Source: CAD feature listing. Evaluate the final solid. Frame: model axes, mm. Face numbers are marked on the shaded views. A direction names the side the tool comes from. Give positions to 0.01 mm unless a question says otherwise; leave off trailing zeros. Order: outer loops, then holes, each group sorted by start corner. A loop starts at its lowest first (then second) coordinate and runs counter-clockwise, first axis right, second up. Notation, with made-up numbers: (-24, -14.5) -> (21, -14.5) arc R15 ccw to (21, -5.5) -> close; hole circle Ø9 at (26.25, 22). An arc over 180 degrees is marked (long way). Answer in a Markdown table with one row per item.
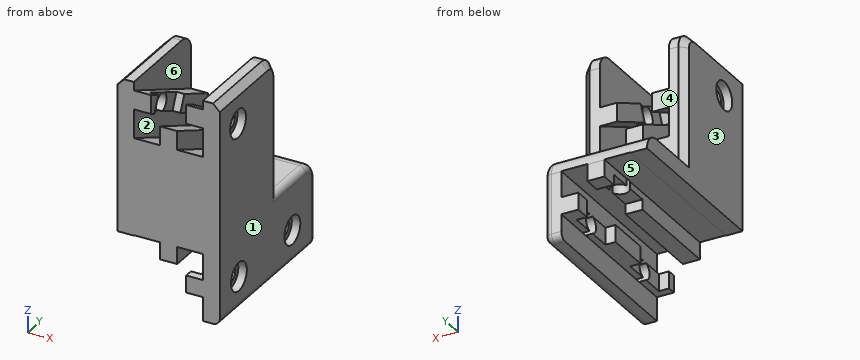
```python
from build123d import *

# Parameters (mm, degrees)
Z_EXTRUSION_MOUNT_W     = 30
Z_EXTRUSION_MOUNT_H     = 30
BOSS_EXTRUDE1_DEPTH     = 50
CUT_EXTRUDE1_DEPTH      = 50
SKETCH3_W               = 30
SKETCH3_H               = 5.505679799
CUT_EXTRUDE3_DEPTH      = 50
SKETCH4_W               = 30
SKETCH4_H               = 30
BOSS_EXTRUDE3_DEPTH     = 40
CUT_EXTRUDE4_DEPTH      = 10
CUT_EXTRUDE4_DEPTH_BACK = 62.479626952
FILLET1_R               = 5
FILLET2_R               = 5
SKETCH11_R              = 2.75
CUT_EXTRUDE14_DEPTH     = 30
SKETCH22_R              = 4.15
CUT_EXTRUDE17_DEPTH     = 2.5
CUT_EXTRUDE18_START     = -2.5
SKETCH23_R              = 4.15
CUT_EXTRUDE18_DEPTH     = 2.5
FILLET4_R               = 2
SKETCH24_W              = 4.875
SKETCH24_H              = 19.494320201
CUT_EXTRUDE19_DEPTH     = 76.828754441
SKETCH25_R              = 2.625
CUT_EXTRUDE20_DEPTH     = 81.156097709
SKETCH26_R              = 4.15
CUT_EXTRUDE21_DEPTH     = 2.5
SKETCH27_R              = 2.625
CUT_EXTRUDE23_DEPTH     = 66.76473219
SKETCH28_R              = 4.15
CUT_EXTRUDE24_DEPTH     = 2.5
SKETCH29_W              = 10
SKETCH29_H              = 15
CUT_EXTRUDE25_DEPTH     = 3
SKETCH31_W              = 10
SKETCH31_H              = 15
CUT_EXTRUDE27_DEPTH     = 3
SKETCH33_W              = 20.25
SKETCH33_H              = 10.783419854
CUT_EXTRUDE29_DEPTH     = 62.479626952
CUT_EXTRUDE30_DEPTH     = 7.5
CHAMFER1_SIZE           = 2
FILLET5_R               = 2


with BuildPart() as part:
    # Z extrusion mount → Boss-Extrude1 (new body)
    with BuildSketch(Plane(origin=(0, 0, 0), x_dir=(1, 0, 0), z_dir=(0, 1, 0))):
        Rectangle(Z_EXTRUSION_MOUNT_W, Z_EXTRUSION_MOUNT_H)
    extrude(amount=BOSS_EXTRUDE1_DEPTH)

    # Sketch2 → Cut-Extrude1 (cut)
    with BuildSketch(Plane(origin=(0, 50, 0), x_dir=(1, 0, 0), z_dir=(0, 1, 0))):
        Polygon((-10.125, 10.125), (-10.125, -10.125), (-2.5, -10.125), (-2.5, -5.125), (2.5, -5.125), (2.5, -10.125), (10.125, -10.125), (10.125, -2.5), (5.125, -2.5), (5.125, 2.5), (10.125, 2.5), (10.125, 10.125), align=None)
    extrude(amount=-CUT_EXTRUDE1_DEPTH, mode=Mode.SUBTRACT)

    # Sketch3 → Cut-Extrude3 (cut)
    with BuildSketch(Plane(origin=(0, 50, 0), x_dir=(1, 0, 0), z_dir=(0, 1, 0))):
        with Locations((0, 12.247160101)):
            Rectangle(SKETCH3_W, SKETCH3_H)
    extrude(amount=-CUT_EXTRUDE3_DEPTH, mode=Mode.SUBTRACT)

    # Sketch4 → Boss-Extrude3 (add)
    with BuildSketch(Plane.XY.offset(15)):
        with Locations((0, 15)):
            Rectangle(SKETCH4_W, SKETCH4_H)
    extrude(amount=BOSS_EXTRUDE3_DEPTH)

    # Sketch12 → Cut-Extrude4 (cut, two sides: drawn at the far end of the back side and taken through both)
    with BuildSketch(Plane(origin=(-15, 30, 35), x_dir=(-1, 0, 0), z_dir=(0, 0.9063077870366478, -0.42261826174070405)).offset(-CUT_EXTRUDE4_DEPTH_BACK)):
        Polygon((-25.051676804, -1.850953689), (-25.051676804, -9.461830913), (-17.412554028, -9.461830913), (-17.412554028, -4.461830913), (-12.412554028, -4.461830913), (-12.412554028, -9.461830913), (-4.801676804, -9.461830913), (-4.801676804, -1.822708137), (-9.801676804, -1.822708137), (-9.801676804, 3.177291863), (-4.801676804, 3.177291863), (-4.801676804, 10.788169087), (-12.440799581, 10.788169087), (-12.440799581, 5.788169087), (-17.440799581, 5.788169087), (-17.440799581, 10.788169087), (-25.051676804, 10.788169087), (-25.051676804, 3.149046311), (-20.051676804, 3.149046311), (-20.051676804, -1.850953689), align=None)
    extrude(amount=CUT_EXTRUDE4_DEPTH + CUT_EXTRUDE4_DEPTH_BACK, mode=Mode.SUBTRACT)

    # Fillet1
    fillet1_edges = [part.edges().sort_by_distance(p)[0] for p in [
        (0, 30, 55),
    ]]
    fillet(fillet1_edges, radius=FILLET1_R)

    # Fillet2
    # the kernel refuses this fillet: 5 mm, written as the material it takes off along each edge
    with BuildSketch(Plane(origin=(-27.5, 50, 15), x_dir=(0, -1, 0), z_dir=(1, 0, 0))) as fillet2_piece_1:
        with BuildLine():
            CenterArc((FILLET2_R, FILLET2_R), FILLET2_R, 180, 90)
            Line((0, FILLET2_R), (0, 0))
            Line((0, 0), (FILLET2_R, 0))
        make_face()
    extrude(amount=55, mode=Mode.SUBTRACT)

    # Sketch11 → Cut-Extrude14 (cut)
    with BuildSketch(Plane.ZY.offset(15)):
        with Locations((45, 9.554930795)):
            Circle(SKETCH11_R)
    extrude(amount=-CUT_EXTRUDE14_DEPTH, mode=Mode.SUBTRACT)

    # Sketch22 → Cut-Extrude17 (cut)
    with BuildSketch(Plane(origin=(15, 0, 0), x_dir=(0, 0, -1), z_dir=(1, 0, 0))):
        with Locations((-45, 9.554930795)):
            Circle(SKETCH22_R)
    extrude(amount=-CUT_EXTRUDE17_DEPTH, mode=Mode.SUBTRACT)

    # Sketch23 → Cut-Extrude18 (cut)
    with BuildSketch(Plane.ZY.offset(15).offset(CUT_EXTRUDE18_START)):
        with Locations(Location((45, 9.554930795, 0), (0, 0, 180))):
            Circle(SKETCH23_R)
    extrude(amount=CUT_EXTRUDE18_DEPTH, mode=Mode.SUBTRACT)

    # Fillet4
    fillet4_edges = [part.edges().sort_by_distance(p)[0] for p in [
        (15, 50, 0.252839899),
        (15, 48.535533906, 13.535533906),
        (15, 37.5, 15),
    ]]
    fillet(fillet4_edges, radius=FILLET4_R)

    # Sketch24 → Cut-Extrude19 (cut, through all)
    with BuildSketch(Plane(origin=(0, 50, 0), x_dir=(1, 0, 0), z_dir=(0, 1, 0))):
        with Locations((-12.5625, -0.252839899)):
            Rectangle(SKETCH24_W, SKETCH24_H)
    extrude(amount=-CUT_EXTRUDE19_DEPTH, mode=Mode.SUBTRACT)

    # Sketch25 → Cut-Extrude20 (cut, through all)
    with BuildSketch(Plane(origin=(15, 0, 0), x_dir=(0, 0, -1), z_dir=(1, 0, 0))):
        with Locations((-0.005679799, 38)):
            Circle(SKETCH25_R)
        with Locations((-0.005679799, 10)):
            Circle(SKETCH25_R)
    extrude(amount=-CUT_EXTRUDE20_DEPTH, mode=Mode.SUBTRACT)

    # Sketch26 → Cut-Extrude21 (cut)
    with BuildSketch(Plane(origin=(15, 0, 0), x_dir=(0, 0, -1), z_dir=(1, 0, 0))):
        with Locations((-0.005679799, 38)):
            Circle(SKETCH26_R)
        with Locations((-0.005679799, 10)):
            Circle(SKETCH26_R)
    extrude(amount=-CUT_EXTRUDE21_DEPTH, mode=Mode.SUBTRACT)

    # Sketch27 → Cut-Extrude23 (cut, through all)
    with BuildSketch(Plane.XY.offset(15)):
        with Locations((0, 37.5)):
            Circle(SKETCH27_R)
    extrude(amount=-CUT_EXTRUDE23_DEPTH, mode=Mode.SUBTRACT)

    # Sketch28 → Cut-Extrude24 (cut)
    with BuildSketch(Plane.XY.offset(15)):
        with Locations((0, 37.5)):
            Circle(SKETCH28_R)
    extrude(amount=-CUT_EXTRUDE24_DEPTH, mode=Mode.SUBTRACT)

    # Sketch29 → Cut-Extrude25 (cut)
    with BuildSketch(Plane(origin=(0, 0, 5.125), x_dir=(-1, 0, 0), z_dir=(0, 0, -1))):
        with Locations((0, 37.5)):
            Rectangle(SKETCH29_W, SKETCH29_H)
    extrude(amount=-CUT_EXTRUDE25_DEPTH, mode=Mode.SUBTRACT)

    # Sketch31 → Cut-Extrude27 (cut)
    with BuildSketch(Plane.ZY.offset(-5.125)):
        with Locations((0.005679799, 38)):
            Rectangle(SKETCH31_W, SKETCH31_H)
        with Locations((0.005679799, 10)):
            Rectangle(SKETCH31_W, SKETCH31_H)
    extrude(amount=-CUT_EXTRUDE27_DEPTH, mode=Mode.SUBTRACT)

    # Sketch33 → Cut-Extrude29 (cut, through all)
    with BuildSketch(Plane(origin=(-15, 30, 35), x_dir=(-1, 0, 0), z_dir=(0, 0.9063077870366478, -0.42261826174070405))):
        with Locations((-14.926676804, 11.08981557)):
            Rectangle(SKETCH33_W, SKETCH33_H)
    extrude(amount=-CUT_EXTRUDE29_DEPTH, mode=Mode.SUBTRACT)

    # Sketch35 → Cut-Extrude30 (cut, symmetric)
    with BuildSketch(Plane(origin=(0, 0, 0), x_dir=(0, 0, -1), z_dir=(1, 0, 0))):
        Polygon((-37.747378495, 14.475156436), (-45.033706868, 17.825136051), (-52.252621505, 4.634705153), (-44.966293132, 1.284725539), align=None)
    extrude(amount=CUT_EXTRUDE30_DEPTH, both=True, mode=Mode.SUBTRACT)

    # Chamfer1
    chamfer1_edges = [part.edges().sort_by_distance(p)[0] for p in [
        (15, 12.5, 55),
        (15, 28.535533906, 53.535533906),
        (15, 30, 31.5),
        (-15, 12.5, 55),
        (-15, 28.535533906, 53.535533906),
        (-15, 30, 32.5),
    ]]
    chamfer(chamfer1_edges, length=CHAMFER1_SIZE)

    # Fillet5
    fillet5_edges = [part.edges().sort_by_distance(p)[0] for p in [
        (14.414213562, 49.414213562, -9.494320201),
        (15, 24, -9.494320201),
        (11.5625, 50, -9.494320201),
    ]]
    fillet(fillet5_edges, radius=FILLET5_R)


solid = part.part
```
(1) Section query A-A (x = 0). Return the cut outline in (y, z) (3 decimals).
A:
| item | result |
|---|---|
| outline | (0, 5.125) -> (30, 5.125) -> (30, 8.125) -> (34.875, 8.125) -> (34.875, 12.5) -> (33.35, 12.5) -> (33.35, 15) -> (30, 15) -> (30, 30.077) -> (0, 44.066) -> close; (40.125, 8.125) -> (45, 8.125) -> (45, 5.125) -> (50, 5.125) -> (50, 10) arc R5 ccw to (45, 15) -> (41.65, 15) -> (41.65, 12.5) -> (40.125, 12.5) -> close |
(2) Section query D-D (x = -8.5). Return the cut outline in (y, z) (3 decimals).
A:
| item | result |
|---|---|
| outline | (0, 10.125) -> (49.998, 10.125) arc R5 ccw to (45, 15) -> (30, 15) -> (30, 24.56) -> (0, 38.549) -> close; (0, 46.978) -> (7.167, 43.636) arc R2.75 cw (long way) to (10.045, 42.294) -> (30, 32.989) -> (30, 38.506) -> (0, 52.495) -> close |
(3) First-contact query: pin 1 Ø3 at (y, z) = (10, 0.01) entering from -X; pin 2 Ø1.5 at (x, y) = (6.5, 24.5) entering from -Z; pin 3 Ø1.5 at (x, y) = (-6, 17.5) entering from -Z (3 decimals); pin 4 Ø4 at (x, y) = (-0.5, 12) entering from -Z (3 decimals). Flat tips, straight axial feed; report the tip coordinate or a pass-through.
A:
| item | result |
|---|---|
| pin 1 | passes through |
| pin 2 | stops at z = -2.5 |
| pin 3 | stops at z = 10.125 |
| pin 4 | stops at z = 5.125 |
(4) Ray query, probe 1 along X at (y, z) = (17, 6.5) (3 decimals); probe 2 along Y at (x, z) = (-10.5, 45); probe 3 along Z at (x, y) = (-11.25, 3.5). Return the intervals inside material, ascending.
A:
| item | result |
|---|---|
| probe 1 | x = -2.5 to 2.5, 10.125 to 15 |
| probe 2 | y = 0 to 6.8, 12.3 to 30 |
| probe 3 | z = 10 to 55 |
(5) Access query for the marked faces 4, 5 and 6. Directions: +Z, -Z, +X, -X, +Y, -Y. A direction counts if a zero-diameter tool reaches every point of the face in a straight line with its end or side. Return the directions, or none.
A:
| item | result |
|---|---|
| face 4 | +Z, +X, -X, +Y |
| face 5 | -Z, +Y, -Y |
| face 6 | +Z, +Y |
(6) Pull-direction query (X, two-part tool) for the marked faces 1, 2 and 3; classes: +X half, -X half, draft (parallel to the pull), parting line (faces both ways), or undercut.
A:
| item | result |
|---|---|
| face 1 | +X half |
| face 2 | undercut |
| face 3 | -X half |
(7) Section query C-C (y = 43). Return the cut outline in (x, z) (3 decimals), plus the area to 3 significant figures.
A:
| item | result |
|---|---|
| outline | (-15, 10) -> (-10.125, 10) -> (-10.125, 10.125) -> (-2.5, 10.125) -> (-2.5, 8.125) -> (2.5, 8.125) -> (2.5, 10.125) -> (10.125, 10.125) -> (10.125, 2.5) -> (8.125, 2.5) -> (8.125, -2.5) -> (10.125, -2.5) -> (10.125, -9.494) -> (13, -9.494) arc R2 ccw to (15, -7.494) -> (15, 13) arc R2 ccw to (13, 15) -> (-15, 15) -> close |
| area | 261 mm^2 |
(8) Section query B-B (z = 21). Return the cut outline in (x, y), plus the area to 3 significant figures.
A:
| item | result |
|---|---|
| outline | (-15, 0) -> (15, 0) -> (15, 28) -> (13, 30) -> (-13, 30) -> (-15, 28) -> close |
| area | 896 mm^2 |
